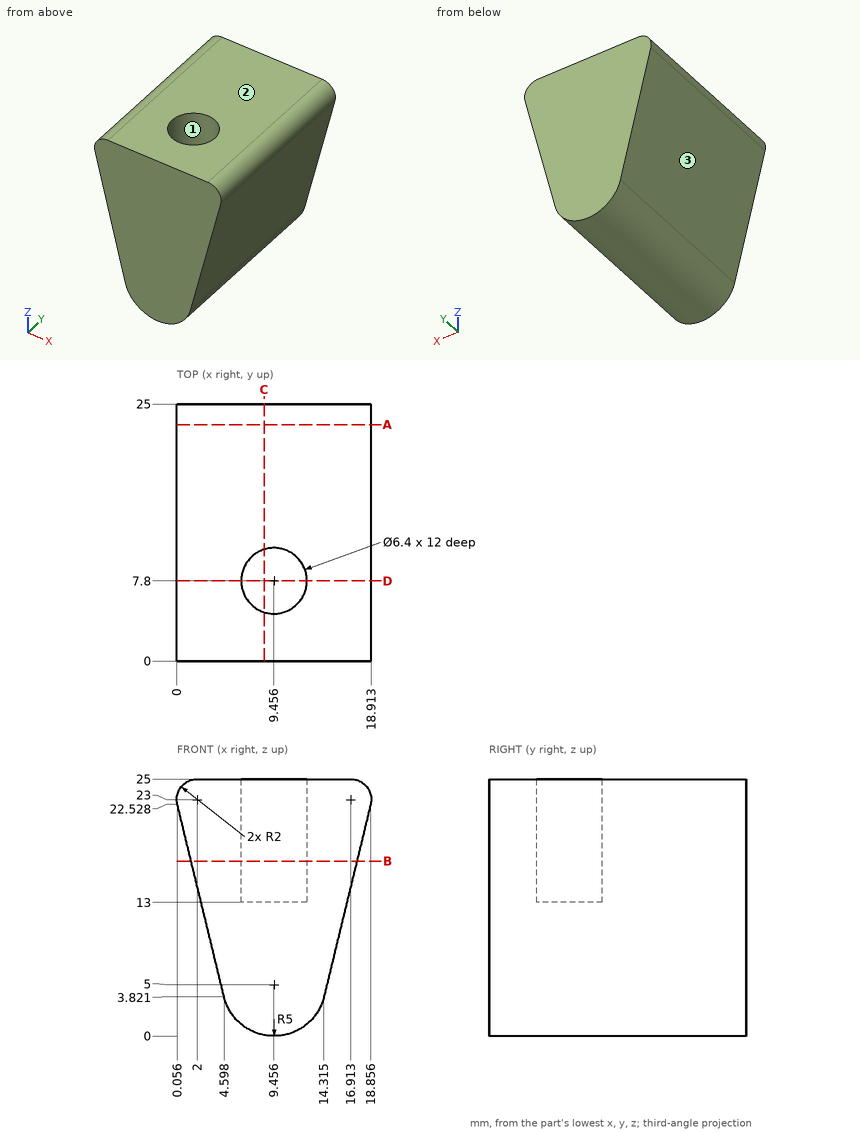
Job drawing, mm, ordinate dimensions from the low corner. One solid piece. Round coordinates to 2 decimals unless told otherwise and drop trailing zeros. Loops run counter-clockwise (first coordinate to the right, second up) from the corner with the lowest first, then second, coordinate; pieces in that order, holes last. Notation, with made-up numbers: M -8.5,77.25 L 24.5,77.25 A31 cw 24.5,111.25 Z; hole C -4,56 d5. An arc over 180 degrees is marked long. Answer as CSV lines item,"result".
1. Wall check: probe 1 along Y at (x, z) = (10, 17.25); probe 2 along Y at (x, z) = (10.5, 20) (1 decimal); probe 3 along X at (y, z) = (6, 2.75). Give the ranges that are in metal, low to high. Write a range as [from, to].
Resolved:
probe 1,"y = [0, 4.65], [10.95, 25]"
probe 2,"y = [0, 4.8], [10.8, 25]"
probe 3,"x = [4.99, 13.92]"
2. Cut at B-B on z = 17. Write the cut outline in (x, y) (1 decimal).
Resolved:
outline,"M 1.4,0 L 17.5,0 L 17.5,25 L 1.4,25 Z; hole C 9.5,7.8 d6.4"
3. Two-plate mould, pull along X, no slides. Class the marked faces 1, 2 and 3: released by +X, released by -X, zero draft, split by the parting line, or undercut.
Resolved:
face 1,"undercut"
face 2,"zero draft"
face 3,"released by -X"
4. Flat gauge pins, fed straight in: P1, Ø2, axis at y = 21.5, z = 6.5, coming from the -X side (1 decimal); P2, Ø6, axis at x = 9.46, y = 7.8, coming from the +Z side; P3, Ø6, axis at y = 15, z = 3, coming from the +X side (1 decimal). Where does each tip first touch, or does it go through?
Resolved:
P1,"stops at x = 3.7"
P2,"stops at z = 13"
P3,"stops at x = 14.8"
5. Cut at D-D on y = 7.8. Write the cut outline in (x, z) (1 decimal).
Resolved:
outline,"M 0.1,22.5 L 4.6,3.8 A5 ccw 14.3,3.8 L 18.9,22.5 A2 ccw 16.9,25 L 12.7,25 L 12.7,13 L 6.3,13 L 6.3,25 L 2,25 A2 ccw Z"
6. Cut at C-C on x = 8.5. Write the cut outline in (y, z).
Resolved:
outline,"M 0,0.09 L 25,0.09 L 25,25 L 10.85,25 L 10.85,13 L 4.75,13 L 4.75,25 L 0,25 Z"
7. Cut at A-A on y = 23. Write the cut outline in (x, z) (1 decimal), then the cut area to 3 significant figures.
Resolved:
outline,"M 0.1,22.5 L 4.6,3.8 A5 ccw 14.3,3.8 L 18.9,22.5 A2 ccw 16.9,25 L 2,25 A2 ccw Z"
area,"339 mm²"
